```python
from build123d import *

# Parameters (mm, degrees)
SKETCH1_R             = 10
BOSS_EXTRUDE1_DEPTH   = 41
CHAMFER1_SIZE         = 0.5
M8_TAPPED_HOLE1_D     = 6.8
M8_TAPPED_HOLE1_DEPTH = 22.25
M8_TAPPED_HOLE1_TIP   = 2.042926105
M8_TAPPED_HOLE2_D     = 6.8
M8_TAPPED_HOLE2_DEPTH = 22.25
M8_TAPPED_HOLE2_TIP   = 2.042926105


with BuildPart() as part:
    # Sketch1 → Boss-Extrude1 (new, symmetric)
    with BuildSketch(Plane(origin=(0, 0, 0), x_dir=(0, 0, -1), z_dir=(1, 0, 0))):
        Circle(SKETCH1_R)
    extrude(amount=BOSS_EXTRUDE1_DEPTH, both=True)

    # Chamfer1
    chamfer1_edges = [part.edges().sort_by_distance(p)[0] for p in [
        (-41, 0, 10),
        (41, 0, 10),
    ]]
    chamfer(chamfer1_edges, length=CHAMFER1_SIZE)

    # M8 Tapped Hole1
    with Locations(Plane(origin=(41, 0, 0), x_dir=(0, 0, -1), z_dir=(1, 0, 0))):
        with Locations((0, 0)):
            Hole(M8_TAPPED_HOLE1_D / 2, depth=M8_TAPPED_HOLE1_DEPTH)
            with Locations((0, 0, -(M8_TAPPED_HOLE1_DEPTH + M8_TAPPED_HOLE1_TIP / 2))):  # 118° drill point
                Cone(0, M8_TAPPED_HOLE1_D / 2, M8_TAPPED_HOLE1_TIP, mode=Mode.SUBTRACT)

    # M8 Tapped Hole2
    with Locations(Plane.ZY.offset(41)):
        with Locations((0, 0)):
            Hole(M8_TAPPED_HOLE2_D / 2, depth=M8_TAPPED_HOLE2_DEPTH)
            with Locations((0, 0, -(M8_TAPPED_HOLE2_DEPTH + M8_TAPPED_HOLE2_TIP / 2))):  # 118° drill point
                Cone(0, M8_TAPPED_HOLE2_D / 2, M8_TAPPED_HOLE2_TIP, mode=Mode.SUBTRACT)


solid = part.part
```
Design review of the part built by this model. Coordinates are the model's own, in mm. A direction names the side the tool comes from. Coordinates: 2 decimals unless noted, no trailing zeros. Write each loop counter-clockwise with the first axis right and the second up, starting at its lowest first coordinate (ties: lowest second). Pieces come first, ordered by that corner, then holes.
1) Insertion check: pin 1 (5 mm diameter, centred on x = -29, y = -3, fed in from -Z); pin 2 (3 mm diameter, centred on x = -11.5, y = -6.5, fed in from +Z); pin 3 (5 mm diameter, centred on x = 0.5, z = -3, fed in from -Y). Each pin has a flat end and moves straight along its axis. Give the tip position at first contact, or say it passes through.
2) Add section A-A (x = -20). Write out the cut boundary in (y, z), plus the area to 3 significant figures.
3) Mouldability with a two-part tool opening along Z and no side actions: class faces 1 (the cylindrical face through (0.57, -9.76, 2.17)), 2 (the cylindrical face through (-29.72, -3.32, 0.74)), 3 (the flat face through (-41, 0, -4)) as +Z half, -Z half, draft (parallel to the pull), parting line (faces both ways), or undercut.
4) To check wall thickness, follow L1, parallel to Y at x = 26.5, z = 0; L2, parallel to Z at x = -27.5, y = 2.25; L3, parallel to Z at x = -28.5, y = 2.5. State the ranges of each line that lie inside material, in increasing order.
5) Machinability: for faces 4 (the cylindrical face through (29.72, -3.32, -0.74)), 5 (the conical face through (-17.062, -0.576, -0.128)), which of the approach directions +Z, -Z, +X, -X, +Y, -Y give a long, thin tool a straight path to every point of the face, cutting with its end or side? Answer none if there is none.
Check result:
1. pin 1: stops at z = -9.99
1. pin 2: stops at z = 8.66
1. pin 3: stops at y = -9.99
2. outline: circle Ø20 at (0, 0); hole circle Ø6.8 at (0, 0)
2. area: 278 mm2
3. face 1: parting line
3. face 2: undercut
3. face 3: draft
4. L1: y = -10 to -3.4, 3.4 to 10
4. L2: z = -9.74 to -2.55, 2.55 to 9.74
4. L3: z = -9.68 to -2.3, 2.3 to 9.68
5. face 4: +X
5. face 5: -X
